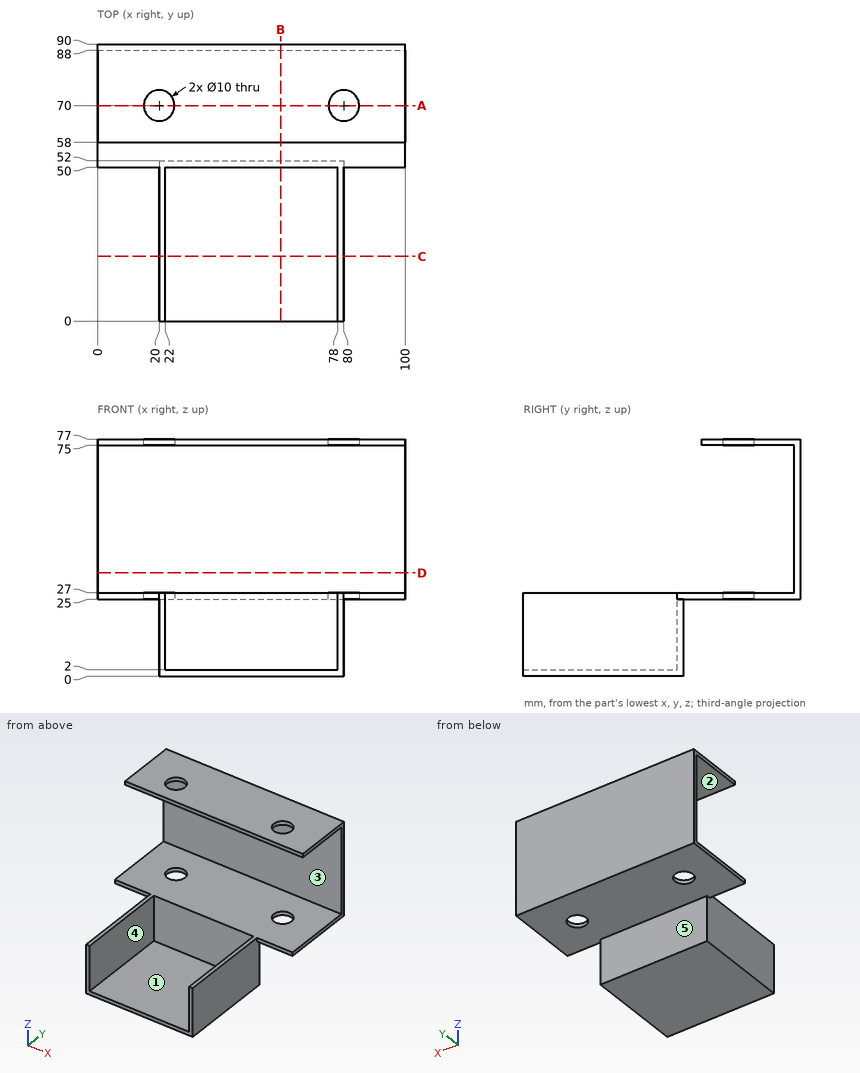
Part print with two shaded views. Sizes in mm from the minimum x, y, z corner. A direction names the side the tool comes from. Round coordinates to 2 decimals unless told otherwise and drop trailing zeros. Order: outer loops, then holes, each group sorted by start corner. A loop starts at its lowest first (then second) coordinate and runs counter-clockwise, first axis right, second up. Notation, with made-up numbers: M -33.75,87 L -24.75,87 A31 ccw -24.75,123 Z; hole C 78.25,9.5 d5. An arc over 180 degrees is marked long. Use CSV: the item, a comma, the result in double quotes. Start each with the question number.
(1) Tool access for the marked faces 3, 4 and 5: list every direction of +Z, -Z, +X, -X, +Y, -Y with a clear straight run to the whole face (end or side of a thin tool).
(2) Drill centre lines: probe 1 along X at (y, z) = (16, 18); probe 2 along Y at (x, z) = (80, 76.65); probe 3 along Z at (x, y) = (41, 58.5). Where is each one in solid material? Low to high.
(3) Mould opens along X. For the marked faces 1 and 2 say: +X half, -X half, draft (parallel to the pull), parting line (faces both ways), or undercut.
(4) Cut at A-A on y = 70. List the corners of the cut face in (x, z).
(5) Cut at B-B on x = 59.5. List the corners of the cut face in (y, z).
(6) Flat gauge pins, fed straight in: P1, Ø2, axis at y = 44.5, z = 8.5, coming from the +X side; P2, Ø24, axis at x = 47.5, z = 51.5, coming from the -Y side; P3, Ø3, axis at y = 46.5, z = 18, coming from the -X side; P4, Ø9, axis at x = 80, y = 70, coming from the +Z side. Where does each tip first touch, or does it go through?
(7) Cut at D-D on z = 33.5. List the corners of the cut face in (x, y).
(8) Cut at C-C on y = 21. List the corners of the cut face in (x, z).
Findings:
1,face 3,"+X, -X, -Y"
1,face 4,"+Z, -Y"
1,face 5,"-Z, +X, -X, +Y"
2,probe 1,"x = 20 to 22, 78 to 80"
2,probe 2,"y = 58 to 65, 75 to 90"
2,probe 3,"z = 25 to 27, 75 to 77"
3,face 1,"undercut"
3,face 2,"draft"
4,outline,"M 0,25 L 15,25 L 15,27 L 0,27 Z; M 0,75 L 15,75 L 15,77 L 0,77 Z; M 25,25 L 75,25 L 75,27 L 25,27 Z; M 25,75 L 75,75 L 75,77 L 25,77 Z; M 85,25 L 100,25 L 100,27 L 85,27 Z; M 85,75 L 100,75 L 100,77 L 85,77 Z"
5,outline,"M 0,0 L 52,0 L 52,25 L 90,25 L 90,77 L 58,77 L 58,75 L 88,75 L 88,27 L 50,27 L 50,2 L 0,2 Z"
6,P1,"stops at x = 80"
6,P2,"stops at y = 88"
6,P3,"stops at x = 20"
6,P4,"passes through"
7,outline,"M 0,88 L 100,88 L 100,90 L 0,90 Z"
8,outline,"M 20,0 L 80,0 L 80,27 L 78,27 L 78,2 L 22,2 L 22,27 L 20,27 Z"
